from build123d import *

# Parameters (mm, degrees)
EXTRUDE_1_DEPTH     = 60
SKETCH_2_W          = 40
SKETCH_2_H          = 130
CUT_EXTRUDE_1_DEPTH = 136
SKETCH_3_W          = 100
SKETCH_3_H          = 140
CUT_EXTRUDE_2_DEPTH = 49
SKETCH_4_R          = 4
CUT_EXTRUDE_3_DEPTH = 198


with BuildPart() as part:
    # 草图1 → 凸台-拉伸1 (new body)
    with BuildSketch(Plane.XY):
        Polygon((-100, 75), (100, 75), (100, 70), (60, 70), (60, -70), (100, -70), (100, -75), (-100, -75), (-100, -70), (-60, -70), (-60, 70), (-100, 70), align=None)
    extrude(amount=EXTRUDE_1_DEPTH)

    # 草图2 → 切除-拉伸1 (cut)
    with BuildSketch(Plane(origin=(60, 0, 0), x_dir=(0, 0, -1), z_dir=(1, 0, 0))):
        with Locations((-31.130418395, 0.098831956)):
            Rectangle(SKETCH_2_W, SKETCH_2_H)
    extrude(amount=-CUT_EXTRUDE_1_DEPTH, mode=Mode.SUBTRACT)

    # 草图3 → 切除-拉伸2 (cut)
    with BuildSketch(Plane.XY.offset(60)):
        Rectangle(SKETCH_3_W, SKETCH_3_H)
    extrude(amount=-CUT_EXTRUDE_2_DEPTH, mode=Mode.SUBTRACT)

    # 草图4 → 切除-拉伸3 (cut)
    with BuildSketch(Plane.XZ.offset(75)):
        with Locations(Location((-80, 30, 0), (0, 0, 270))):
            Circle(SKETCH_4_R)
        with Locations(Location((80, 30, 0), (0, 0, 270))):
            Circle(SKETCH_4_R)
    extrude(amount=-CUT_EXTRUDE_3_DEPTH, mode=Mode.SUBTRACT)


solid = part.part
Here's how the part is built. I have some questions about the finished solid (model axes, mm). A direction names the side the tool comes from. Give positions to 0.01 mm unless a question says otherwise; leave off trailing zeros. Order: outer loops, then holes, each group sorted by start corner. A loop starts at its lowest first (then second) coordinate and runs counter-clockwise, first axis right, second up. Notation, with made-up numbers: (-25, -23) -> (-14, -23) arc R28 cw to (-14, 13) -> close; hole circle Ø1 at (-3.75, 88.5). An arc over 180 degrees is marked (long way). One line per item, written item: value. Start each with the question number.
1. Imagine slicing it at A-A, the plane y = 53. List the corners of the cut face in (x, z) for me, plus the area to 3 significant figures.
2. Imagine slicing it at B-B, the plane z = 13.5. List the corners of the cut face in (x, y) for me.
3. Imagine slicing it at C-C, the plane x = 80. List the corners of the cut face in (y, z) for me, plus the area to 3 significant figures.
4. Imagine slicing it at D-D, the plane x = -72. List the corners of the cut face in (y, z) for me.
5. I need wall thicknesses on probe 1 along X at (y, z) = (73.25, 30); probe 2 along Z at (x, y) = (57, -62); probe 3 along Y at (x, z) = (17, 31.5). Which ranges of each line are inside material? Lowest first, please. Write a range as from..to.
6. Will these pins go through, and if not, where does the flat tip stop? pin 1 Ø5 at (x, z) = (-80, 30) entering from +Y; pin 2 Ø10 at (x, y) = (-23.5, 31) entering from +Z; pin 3 Ø3 at (x, y) = (-42.5, -57.5) entering from -Z.
7. For faces 5 (the face through (60, 0, 8)), 6 (the face through (-85, -70, 30)), 7 (the face through (76.095, 72.465, 30.867)), 8 (the face through (-55, -1, 11.13)), 9 (the face through (-50, 0, 54)), which set-ups out of +Z, -Z, +X, -X, +Y, -Y let a thin tool reach every point of the face, with its end or its side?
8. We'd pull the mould along X, two halves only. Please class faces 1 (the face through (76.095, -72.535, 30.867)), 2 (the face through (50, 0, 54)), 3 (the face through (-60, 0, 8)), 4 (the face through (-55, -64.901, 31)): released by +X, released by -X, zero draft, split by the parting line, or undercut.
Values follow:
1. outline: (-60, 0) -> (60, 0) -> (60, 11.13) -> (50, 11.13) -> (50, 11) -> (-50, 11) -> (-50, 11.13) -> (-60, 11.13) -> close; (-60, 51.13) -> (-50, 51.13) -> (-50, 60) -> (-60, 60) -> close; (50, 51.13) -> (60, 51.13) -> (60, 60) -> (50, 60) -> close
1. area: 1,500 mm2
2. outline: (-100, -75) -> (100, -75) -> (100, -70) -> (60, -70) -> (60, -64.9) -> (50, -64.9) -> (50, -70) -> (-50, -70) -> (-50, -64.9) -> (-60, -64.9) -> (-60, -70) -> (-100, -70) -> close; (-100, 70) -> (-60, 70) -> (-60, 65.1) -> (-50, 65.1) -> (-50, 70) -> (50, 70) -> (50, 65.1) -> (60, 65.1) -> (60, 70) -> (100, 70) -> (100, 75) -> (-100, 75) -> close
3. outline: (-75, 0) -> (-70, 0) -> (-70, 26) -> (-75, 26) -> close; (-75, 34) -> (-70, 34) -> (-70, 60) -> (-75, 60) -> close; (70, 0) -> (75, 0) -> (75, 26) -> (70, 26) -> close; (70, 34) -> (75, 34) -> (75, 60) -> (70, 60) -> close
3. area: 520 mm2
4. outline: (-75, 0) -> (-70, 0) -> (-70, 60) -> (-75, 60) -> close; (70, 0) -> (75, 0) -> (75, 60) -> (70, 60) -> close
5. probe 1: x = -100..-84, -76..76, 84..100
5. probe 2: z = 0..11.13, 51.13..60
5. probe 3: y = -75..-70, 70..75
6. pin 1: passes through
6. pin 2: stops at z = 11
6. pin 3: stops at z = 0
7. face 5: +Z, -Z, +X
7. face 6: +Z, -Z, -X
7. face 7: +Y, -Y
7. face 8: +X, -X
7. face 9: +Z
8. face 1: undercut
8. face 2: undercut
8. face 3: released by -X
8. face 4: zero draft
